Verification items for this drawing (mm, ordinates from the low corner). A direction names the side the tool comes from. Coordinates: 2 decimals unless noted, no trailing zeros. Write each loop counter-clockwise with the first axis right and the second up, starting at its lowest first coordinate (ties: lowest second). Pieces come first, ordered by that corner, then holes. Notation, with made-up numbers: (-26.75, 52.5) -> (-13.75, 52.5) arc R21 ccw to (-13.75, 62.5) -> close; hole circle Ø7 at (20.5, 79.5). An arc over 180 degrees is marked (long way). One line per item, written item: value. Start each with the question number.
1) Sectioned sample at B-B on z = 4.75. Enter the section's corners in (x, y).
2) Scan lines: line 1 along Y through (x, z) = (87.5, 13); line 2 along Y through (x, z) = (33, 3.5); line 3 along X through (y, z) = (24, 6.75). Record each from-to range of solid material in increasing order. Write a range as [from, to].
3) Sectioned sample at A-A on z = 11.5. Enter the section's corners in (x, y), plus the area to 3 significant figures.
4) Set-up check for the marked faces 4, 5 and 6: record each of +Z, -Z, +X, -X, +Y, -Y from which the full face is reachable in a straight line by a thin tool's end or side.
5) Gauge pin test, flat ends, axial feed: P1, Ø3.5, axis at x = 12.5, y = 45.5, coming from the +Z side; P2, Ø0.9, axis at x = 12, y = 46, coming from the +Z side. Record the tip position at first contact, or that the pin passes through.
6) Sectioned sample at C-C on x = 48. Enter the section's corners in (y, z), plus the area to 3 significant figures.
7) Sectioned sample at D-D on x = 12.5. Enter the section's corners in (y, z).
8) Draft check along Y on the marked faces 1, 2 and 3. Enter one of: +Y half, -Y half, draft (parallel to the pull), parting line (faces both ways), or undercut.
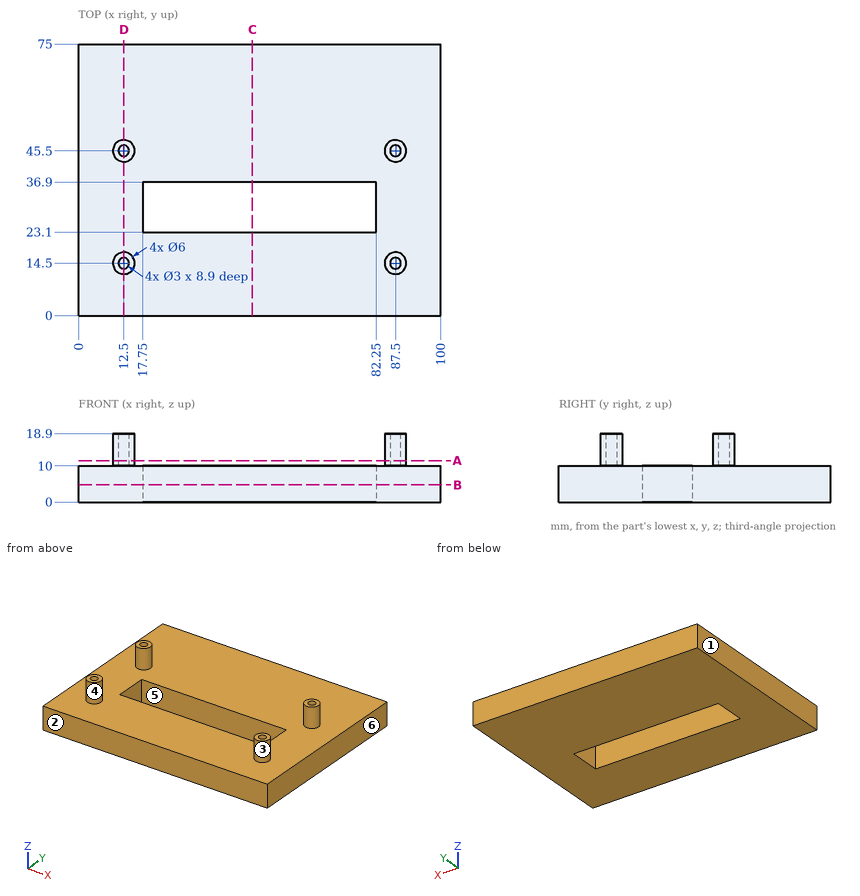
Answers:
1. outline: (0, 0) -> (100, 0) -> (100, 75) -> (0, 75) -> close; hole (17.75, 23.1) -> (82.25, 23.1) -> (82.25, 36.9) -> (17.75, 36.9) -> close
2. line 1: y = [11.5, 13], [16, 17.5], [42.5, 44], [47, 48.5]
2. line 2: y = [0, 23.1], [36.9, 75]
2. line 3: x = [0, 17.75], [82.25, 100]
3. outline: circle Ø6 at (12.5, 14.5); circle Ø6 at (12.5, 45.5); circle Ø6 at (87.5, 14.5); circle Ø6 at (87.5, 45.5); hole circle Ø3 at (12.5, 14.5); hole circle Ø3 at (12.5, 45.5); hole circle Ø3 at (87.5, 14.5); hole circle Ø3 at (87.5, 45.5)
3. area: 84.8 mm2
4. face 4: +Z
4. face 5: +Z, -Z
4. face 6: +Z, -Z, +X, +Y, -Y
5. P1: stops at z = 18.9
5. P2: stops at z = 10
6. outline: (0, 0) -> (23.1, 0) -> (23.1, 10) -> (0, 10) -> close; (36.9, 0) -> (75, 0) -> (75, 10) -> (36.9, 10) -> close
6. area: 612 mm2
7. outline: (0, 0) -> (75, 0) -> (75, 10) -> (48.5, 10) -> (48.5, 18.9) -> (47, 18.9) -> (47, 10) -> (44, 10) -> (44, 18.9) -> (42.5, 18.9) -> (42.5, 10) -> (17.5, 10) -> (17.5, 18.9) -> (16, 18.9) -> (16, 10) -> (13, 10) -> (13, 18.9) -> (11.5, 18.9) -> (11.5, 10) -> (0, 10) -> close
8. face 1: draft
8. face 2: -Y half
8. face 3: undercut
